Job drawing, mm, ordinate dimensions from the low corner. One solid piece. Coordinates: 2 decimals unless noted, no trailing zeros. Loops run counter-clockwise (first coordinate to the right, second up) from the corner with the lowest first, then second, coordinate; pieces in that order, holes last. Notation, with made-up numbers: (-6.5, -19) - (36.5, -19) arc R25 ccw to (36.5, 20) - close; hole circle Ø5 at (77, 53.25). An arc over 180 degrees is marked (long way). Use a Markdown table: item, result. Add a question column.
1) Probe probe 1 along Y at (x, z) = (24, 3.65); probe 2 along Y at (x, z) = (13.75, 1.5) (1 decimal); probe 3 along Z at (x, y) = (29.5, 46). List the from-to ranges inside material, lowest first. Write a range as [from, to].
2) Band-saw the part on B-B (y = 24). Give the cut face in (x, z).
3) Drop flat-ended pins along their axis: P1, Ø1, axis at x = 5, z = 1.5, coming from the -Y side; P2, Ø8, axis at x = 14.5, y = 39.5, coming from the -Z side; P3, Ø3, axis at y = 10, z = 3, coming from the -X side; P4, Ø3, axis at y = 21, z = 4.5, coming from the +X side. Give the stop position or say it passes through.
4) Band-saw the part on A-A (x = 24). Give the cut face in (y, z).
5) Pull direction X, two halves, no side cores. Call the marked faces 1, 2 and 3: +X half, -X half, draft (parallel to the pull), parting line (faces both ways), or undercut.
6) Band-saw the part on C-C (z = 5.4). Give the cut face in (x, y).
7) Band-saw the part on D-D (x = 13.75). Give the cut face in (y, z).
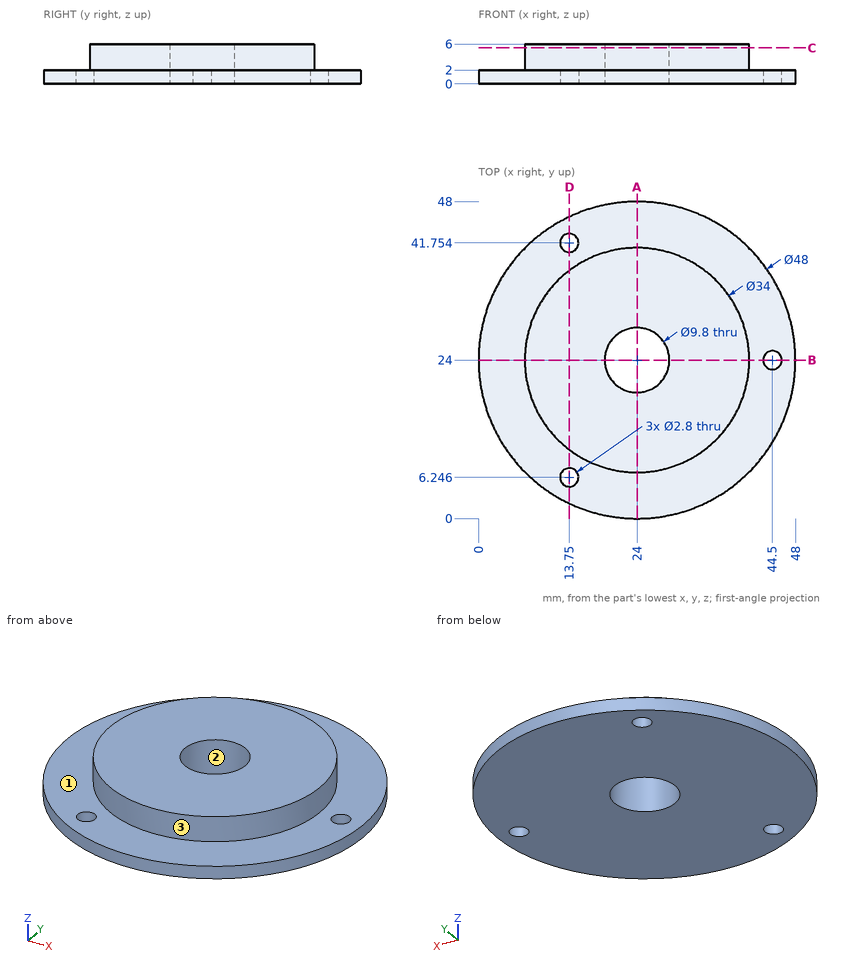
Answer block:
| question | item | result |
|---|---|---|
| 1 | probe 1 | [7, 19.1], [28.9, 41] |
| 1 | probe 2 | [2.3, 4.8], [7.6, 40.4], [43.2, 45.7] |
| 1 | probe 3 | [0, 2] |
| 2 | outline | (0, 0) - (19.1, 0) - (19.1, 6) - (7, 6) - (7, 2) - (0, 2) - close; (28.9, 0) - (43.1, 0) - (43.1, 2) - (41, 2) - (41, 6) - (28.9, 6) - close; (45.9, 0) - (48, 0) - (48, 2) - (45.9, 2) - close |
| 3 | P1 | y = 8.71 |
| 3 | P2 | z = 0 |
| 3 | P3 | x = 3.75 |
| 3 | P4 | x = 40.93 |
| 4 | outline | (0, 0) - (19.1, 0) - (19.1, 6) - (7, 6) - (7, 2) - (0, 2) - close; (28.9, 0) - (48, 0) - (48, 2) - (41, 2) - (41, 6) - (28.9, 6) - close |
| 5 | face 1 | draft |
| 5 | face 2 | undercut |
| 5 | face 3 | parting line |
| 6 | outline | circle Ø34 at (24, 24); hole circle Ø9.8 at (24, 24) |
| 7 | outline | (2.3, 0) - (4.85, 0) - (4.85, 2) - (2.3, 2) - close; (7.65, 0) - (40.35, 0) - (40.35, 2) - (37.56, 2) - (37.56, 6) - (10.44, 6) - (10.44, 2) - (7.65, 2) - close; (43.15, 0) - (45.7, 0) - (45.7, 2) - (43.15, 2) - close |
